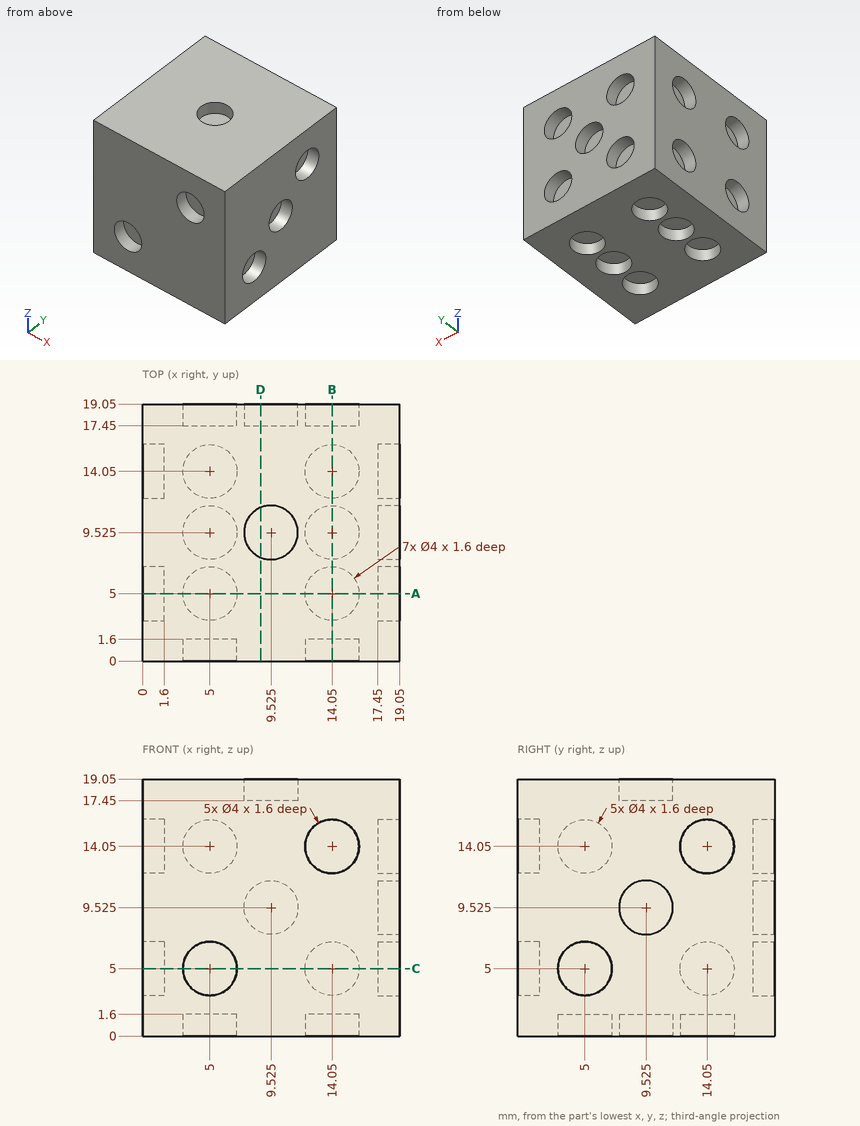
Study the drawing (mm; zero at the part's minimum x, y, z) and answer. Coordinates: 2 decimals unless noted, no trailing zeros. Loops run counter-clockwise (first coordinate to the right, second up) from the corner with the lowest first, then second, coordinate; pieces in that order, holes last. Notation, with made-up numbers: M 39.25,8.5 L 68.25,8.5 A30 ccw 68.25,33.5 Z; hole C 58.5,-37 d7. An arc over 180 degrees is marked long. Answer in a Markdown table with one row per item.
1) Find section A-A (y = 5). Determine the outline of the cut face in (x, z), then the cut area to 3 significant figures.
Answers below:
| item | result |
|---|---|
| outline | M 0,0 L 3,0 L 3,1.6 L 7,1.6 L 7,0 L 12.05,0 L 12.05,1.6 L 16.05,1.6 L 16.05,0 L 19.05,0 L 19.05,3 L 17.45,3 L 17.45,7 L 19.05,7 L 19.05,19.05 L 0,19.05 L 0,16.05 L 1.6,16.05 L 1.6,12.05 L 0,12.05 L 0,7 L 1.6,7 L 1.6,3 L 0,3 Z |
| area | 331 mm^2 |
2) Find section D-D (x = 8.75). Determine the outline of the cut face in (y, z).
Answers below:
| item | result |
|---|---|
| outline | M 0,0 L 19.05,0 L 19.05,7.68 L 17.45,7.68 L 17.45,11.37 L 19.05,11.37 L 19.05,19.05 L 11.37,19.05 L 11.37,17.45 L 7.68,17.45 L 7.68,19.05 L 0,19.05 Z |
3) Find the intervals of material crossed by probe 1 along Y at (x, z) = (5, 0.9) (3 decimals); probe 2 along X at (y, z) = (5, 0.4), in increasing order.
Answers below:
| item | result |
|---|---|
| probe 1 | 0 to 3, 7 to 7.525, 11.525 to 12.05, 16.05 to 19.05 |
| probe 2 | 0 to 3, 7 to 12.05, 16.05 to 19.05 |
4) Find section B-B (x = 14.05). Determine the outline of the cut face in (y, z) (3 decimals), then the cut area to 3 significant figures.
Answers below:
| item | result |
|---|---|
| outline | M 0,0 L 3,0 L 3,1.6 L 7,1.6 L 7,0 L 7.525,0 L 7.525,1.6 L 11.525,1.6 L 11.525,0 L 12.05,0 L 12.05,1.6 L 16.05,1.6 L 16.05,0 L 19.05,0 L 19.05,3 L 17.45,3 L 17.45,7 L 19.05,7 L 19.05,12.05 L 17.45,12.05 L 17.45,16.05 L 19.05,16.05 L 19.05,19.05 L 0,19.05 L 0,16.05 L 1.6,16.05 L 1.6,12.05 L 0,12.05 Z |
| area | 325 mm^2 |
5) Given pin 1 (2 mm diameter, centred on x = 9.5, y = 9, fed in from +Z); pin 2 (3.5 mm diameter, centred on y = 5, z = 14.05, fed in from -X); pin 3 (1.2 mm diameter, centred on y = 9, z = 10.5, fed in from +X); pin 4 (3 mm diameter, centred on x = 14.5, z = 5.5, fed in from +Y), each flat-ended and moving along its own axis, determine where each tip first touches the part or whether it passes through.
Answers below:
| item | result |
|---|---|
| pin 1 | z = 17.45 |
| pin 2 | x = 1.6 |
| pin 3 | x = 17.45 |
| pin 4 | y = 19.05 |
6) Find section C-C (z = 5). Determine the outline of the cut face in (x, y).
Answers below:
| item | result |
|---|---|
| outline | M 0,0 L 3,0 L 3,1.6 L 7,1.6 L 7,0 L 19.05,0 L 19.05,3 L 17.45,3 L 17.45,7 L 19.05,7 L 19.05,19.05 L 16.05,19.05 L 16.05,17.45 L 12.05,17.45 L 12.05,19.05 L 7,19.05 L 7,17.45 L 3,17.45 L 3,19.05 L 0,19.05 L 0,16.05 L 1.6,16.05 L 1.6,12.05 L 0,12.05 L 0,7 L 1.6,7 L 1.6,3 L 0,3 Z |
